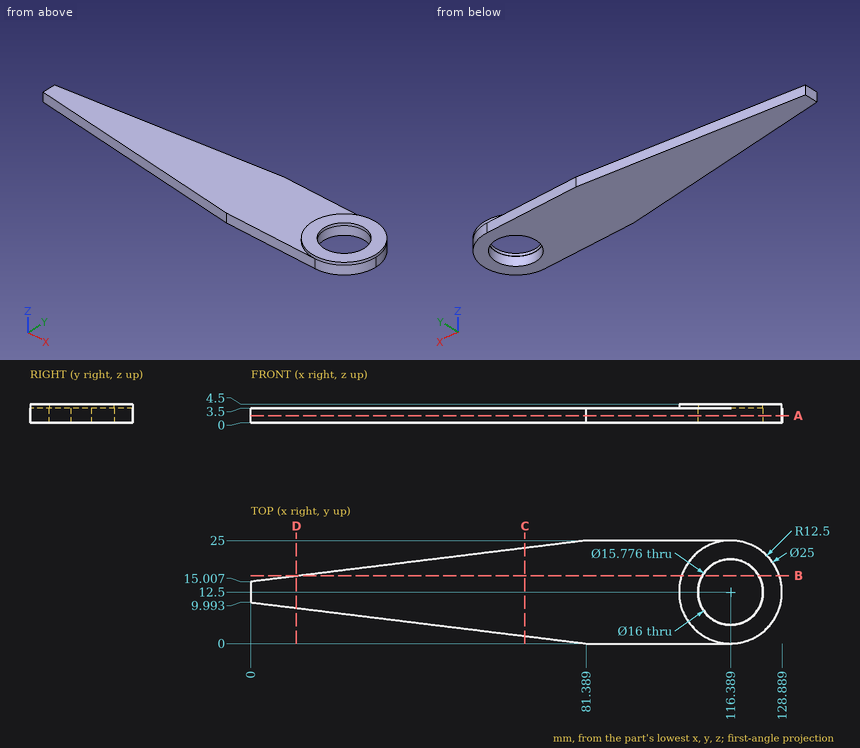
Source: three-view drawing plus pictorial views. Frame: mm from the lowest corner of the part. Give positions to 0.01 mm unless a question says otherwise; leave off trailing zeros. Loops run counter-clockwise (first coordinate to the right, second up) from the corner with the lowest first, then second, coordinate; pieces in that order, holes last. Notation, with made-up numbers: M -8,-12 L 11,-12 A23 ccw 11,7 Z; hole C -28,27 d8. An arc over 180 degrees is marked long. Put each result on its own line as item: value.
Q1. Section B-B (y = 16.5). Return the cut outline in (x, z), and give its area (3 significant figures).
Response values:
outline: M 12.16,0 L 109.46,0 L 109.46,3.5 L 109.59,3.5 L 109.59,4.5 L 104.55,4.5 L 104.55,3.5 L 12.16,3.5 Z; M 123.19,3.5 L 123.32,3.5 L 123.32,0 L 128.23,0 L 128.23,4.5 L 123.19,4.5 Z
area: 368 mm²
Q2. Section D-D (x = 11). Return the cut outline in (y, z), and give its area (3 significant figures).
Response values:
outline: M 8.64,0 L 16.36,0 L 16.36,3.5 L 8.64,3.5 Z
area: 27.0 mm²
Q3. Line query: probe 1 along Z at (x, y) = (51, 7.5); probe 2 along Y at (x, z) = (120, 0.3); probe 3 along X at (y, z) = (11.25, 0.75). Output: solid intervals per line, ascending. Write a range as [from, to].
Response values:
probe 1: z = [0, 3.5]
probe 2: y = [0.53, 5.36], [19.64, 24.47]
probe 3: x = [0, 108.49], [124.29, 128.83]
Q4. Section C-C (x = 66.5). Return the cut outline in (y, z), and give its area (3 significant figures).
Response values:
outline: M 1.83,0 L 23.17,0 L 23.17,3.5 L 1.83,3.5 Z
area: 74.7 mm²
Q5. Section A-A (z = 1.65). Return the cut outline in (x, y), and give its area (3 significant figures).
Response values:
outline: M 0,9.99 L 81.39,0 L 116.39,0 A12.5 ccw 128.89,12.5 A12.5 ccw 116.39,25 L 81.39,25 L 0,15.01 Z; hole C 116.39,12.5 d16
area: 2,140 mm²
Q6. Pin query (flat end, axial travel): P1, Ø12.5, axis at x = 80.5, y = 7, coming from the +Z side; P2, Ø1, axis at y = 22.5, z = 4, coming from the +X side. Return the tip coordinate at first contact, or that it passes through.
Response values:
P1: stops at z = 3.5
P2: stops at x = 124.51
